Verification items for the finished model (mm, model axes). A direction names the side the tool comes from. Give positions to 0.01 mm unless a question says otherwise; leave off trailing zeros. Order: outer loops, then holes, each group sorted by start corner. A loop starts at its lowest first (then second) coordinate and runs counter-clockwise, first axis right, second up.
from build123d import *

# Parameters (mm, degrees)
SKETCH1_W                                     = 230
SKETCH1_H                                     = 123
SKETCH1_W_2                                   = 206
SKETCH1_H_2                                   = 99
BOSS_EXTRUDE1_DEPTH                           = 4
SKETCH2_W                                     = 230
SKETCH2_H                                     = 4
BOSS_EXTRUDE2_DEPTH                           = 6
BOSS_EXTRUDE3_DEPTH                           = 5
FILLET1_R                                     = 15
BOSS_EXTRUDE4_DEPTH                           = 4
FILLET2_R                                     = 5
FILLET3_R                                     = 3
CSK_FOR_4_FLAT_HEAD_MACHINE_SCREW1_AT_2_COUNT = 2
CSK_FOR_4_FLAT_HEAD_MACHINE_SCREW1_AT_2_PITCH = 30
CSK_FOR_4_FLAT_HEAD_MACHINE_SCREW1_AT_3_COUNT = 2
CSK_FOR_4_FLAT_HEAD_MACHINE_SCREW1_AT_3_PITCH = 225.008888713
CSK_FOR_4_FLAT_HEAD_MACHINE_SCREW1_AT_4_COUNT = 2
CSK_FOR_4_FLAT_HEAD_MACHINE_SCREW1_AT_4_PITCH = 223


with BuildPart() as part:
    # Sketch1 → Boss-Extrude1 (new body)
    with BuildSketch(Plane.XY):
        Rectangle(SKETCH1_W, SKETCH1_H)
        Rectangle(SKETCH1_W_2, SKETCH1_H_2, mode=Mode.SUBTRACT)
    extrude(amount=BOSS_EXTRUDE1_DEPTH)

    # Sketch2 → Boss-Extrude2 (add)
    with BuildSketch(Plane(origin=(0, 61.5, 0), x_dir=(1, 0, 0), z_dir=(0, 1, 0))):
        Polygon((-115, 10), (-115, 0), (115, 0), (115, 10), (115, 93), (105, 93), (105, 10), (-105, 10), (-105, 93), (-115, 93), align=None)
        with Locations((0, -2)):
            Rectangle(SKETCH2_W, SKETCH2_H)
    boss_extrude2 = extrude(amount=BOSS_EXTRUDE2_DEPTH)

    # Mirror1: Boss-Extrude2 across plane
    add(boss_extrude2.mirror(Plane.ZX))

    # Sketch3 → Boss-Extrude3 (add)
    with BuildSketch(Plane.ZY.offset(115)):
        Polygon((-93, 61.5), (0, 61.5), (0, -61.5), (-93, -61.5), (-93, -67.5), (4, -67.5), (4, 67.5), (-93, 67.5), align=None)
        Polygon((0, 61.5), (-25, 61.5), (-21.666666667, 57.5), (0, 31.5), align=None)
        Polygon((0, -61.5), (0, -31.5), (-21.666666667, -57.5), (-25, -61.5), align=None)
        Polygon((-21.666666667, 57.5), (-25, 61.5), (-93, 61.5), (-93, 57.5), align=None)
        Polygon((-25, -61.5), (-21.666666667, -57.5), (-93, -57.5), (-93, -61.5), align=None)
    boss_extrude3 = extrude(amount=BOSS_EXTRUDE3_DEPTH)

    # Mirror2: Boss-Extrude3 across plane
    add(boss_extrude3.mirror(Plane(origin=(0, 0, 0), x_dir=(0, 0, 1), z_dir=(1, 0, 0))))

    # Fillet1
    fillet1_edges = [part.edges().sort_by_distance(p)[0] for p in [
        (117.5, 57.5, -21.666666667),
        (117.5, -57.5, -21.666666667),
        (117.5, -31.5, 0),
        (117.5, 31.5, 0),
        (-103, -49.5, 2),
        (103, -49.5, 2),
        (103, 49.5, 2),
        (-103, 49.5, 2),
        (105, 64.5, -10),
        (-105, 64.5, -10),
        (-105, -64.5, -10),
        (105, -64.5, -10),
        (-117.5, 57.5, -21.666666667),
        (-117.5, 31.5, 0),
        (-117.5, -31.5, 0),
        (-117.5, -57.5, -21.666666667),
    ]]
    fillet(fillet1_edges, radius=FILLET1_R)

    # Sketch4 → Boss-Extrude4 (add, symmetric)
    with BuildSketch(Plane(origin=(0, 0, 0), x_dir=(1, 0, 0), z_dir=(0, 1, 0))):
        Polygon((-120, 96.464101615), (-120, 0), (-116.5, 0), (-116.5, 90), (-110.5, 93.464101615), (-110.5, 96.464101615), align=None)
    extrude(amount=BOSS_EXTRUDE4_DEPTH, both=True)

    # Fillet2
    fillet2_edges = [part.edges().sort_by_distance(p)[0] for p in [
        (-118.25, 4, 0),
        (-118.25, -4, 0),
    ]]
    fillet(fillet2_edges, radius=FILLET2_R)

    # Fillet3
    fillet3_edges = [part.edges().sort_by_distance(p)[0] for p in [
        (120, 62.5, -93),
        (120, -62.5, -93),
        (105, 64.5, -93),
        (-120, 0, -96.464101615),
        (-105, 64.5, -93),
        (-105, -64.5, -93),
        (105, -64.5, -93),
        (-120, -62.5, -93),
        (-120, 62.5, -93),
    ]]
    fillet(fillet3_edges, radius=FILLET3_R)

    # Sketch6 → CSK for #4 Flat Head Machine Screw1 (revolve, cut)
    with BuildSketch(Plane(origin=(111.5, 61.5, -68), x_dir=(0, 0, -1), z_dir=(1, 0, 0))):
        Polygon((0, 0), (0, 6), (1.63195, 6), (1.63195, 2.409835609), (2.857501397, 1), (2.857501397, 0), align=None)
    csk_for_4_flat_head_machine_screw1 = revolve(axis=Axis((111.5, 55.15, -68), (0, 1, 0)), mode=Mode.SUBTRACT)

    # CSK for #4 Flat Head Machine Screw1 at 2: CSK for #4 Flat Head Machine Screw1 ×2
    with Locations(*[(0, 0, i * CSK_FOR_4_FLAT_HEAD_MACHINE_SCREW1_AT_2_PITCH) for i in range(1, CSK_FOR_4_FLAT_HEAD_MACHINE_SCREW1_AT_2_COUNT)]):
        add(csk_for_4_flat_head_machine_screw1, mode=Mode.SUBTRACT)

    # CSK for #4 Flat Head Machine Screw1 at 3: CSK for #4 Flat Head Machine Screw1 ×2
    with Locations(*[Vector(-0.9910719584243963, 0, 0.13332806615574816) * (i * CSK_FOR_4_FLAT_HEAD_MACHINE_SCREW1_AT_3_PITCH) for i in range(1, CSK_FOR_4_FLAT_HEAD_MACHINE_SCREW1_AT_3_COUNT)]):
        add(csk_for_4_flat_head_machine_screw1, mode=Mode.SUBTRACT)

    # CSK for #4 Flat Head Machine Screw1 at 4: CSK for #4 Flat Head Machine Screw1 ×2
    with Locations(*[(-i * CSK_FOR_4_FLAT_HEAD_MACHINE_SCREW1_AT_4_PITCH, 0, 0) for i in range(1, CSK_FOR_4_FLAT_HEAD_MACHINE_SCREW1_AT_4_COUNT)]):
        add(csk_for_4_flat_head_machine_screw1, mode=Mode.SUBTRACT)


solid = part.part
(1) Section check A-A, the plane y = -15. Enter the section's corners in (x, z), then the cut area to 3 significant figures.
Solved:
outline: (-120, 0) - (-103, 0) - (-103, 4) - (-120, 4) - close; (103, 0) - (120, 0) - (120, 4) - (103, 4) - close
area: 136 mm2
(2) Release check for a two-part mould opening along Z. For faces 1 (the cylindrical face through (-117.54, -56.12, -22.41)), 2 (the flat face through (120, 0, 2)), 3 (the flat face through (-113.54, 0.06, -91.71)), 4 (the cylindrical face through (114.035, 61.993, -69.319)) record: pulls with the +Z half, pulls with the -Z half, needs draft (parallel to the pull), parting line crosses it, or undercut.
Solved:
face 1: pulls with the -Z half
face 2: needs draft
face 3: undercut
face 4: undercut
(3) Go/stop test with flat-tipped pins: pin 1 (4 mm diameter, centred on x = 111.5, z = -38, fed in from +Y); pin 2 (6 mm diameter, centred on x = -9, y = -45, fed in from -Z) (3 decimals); pin 3 (0.9 mm diameter, centred on y = -1.5, z = -94.5, fed in from +X); pin 4 (6.5 mm diameter, centred on x = 40, y = -66, fed in from -Z). Record where each tip stops, or that it passes through.
Solved:
pin 1: stops at y = 67.5
pin 2: passes through
pin 3: stops at x = -110.5
pin 4: stops at z = -10
(4) Scan lines: line 1 (X direction, y = 65.5, z = -68); line 2 (Z direction, x = 111.5, y = 62.25); line 3 (Z direction, x = 111.5, y = 66.35). Record each from-to range of solid material in increasing order.
Solved:
line 1: x = -120 to -113.13, -109.87 to -105, 105 to 109.87, 113.13 to 120
line 2: z = -93 to -70.86, -65.14 to -40.86, -35.14 to 4
line 3: z = -93 to -69.63, -66.37 to -39.63, -36.37 to 4
(5) Section check B-B, the plane x = -59. Enter the section's corners in (y, z).
Solved:
outline: (-67.5, -10) - (-61.5, -10) - (-61.5, 0) - (-49.5, 0) - (-49.5, 4) - (-67.5, 4) - close; (49.5, 0) - (61.5, 0) - (61.5, -10) - (67.5, -10) - (67.5, 4) - (49.5, 4) - close
(6) Set-up check for faces 5 (the flat face through (-113, 64, -93)), 6 (the cylindrical face through (117.54, -31.24, -0.92)), 7 (the cylindrical face through (100.72, 64.54, -14.51)), 8 (the cylindrical face through (-108.965, 61.993, -39.319)), 9 (the cylindrical face through (-98.72, 44.99, 2.03)): record each of +Z, -Z, +X, -X, +Y, -Y from which the full face is reachable in a straight line by a thin tool's end or side.
Solved:
face 5: -Z, +X, -X, +Y
face 6: -Z, +X, -X
face 7: -Z, +Y, -Y
face 8: none
face 9: +Z, -Z
(7) Section check C-C, the plane z = -75.5. Enter the section's corners in (x, y).
Solved:
outline: (-120, -67.5) - (-105, -67.5) - (-105, -61.5) - (-115, -61.5) - (-115, -57.5) - (-120, -57.5) - close; (-120, -4) - (-116.5, -4) - (-116.5, 4) - (-120, 4) - close; (-120, 57.5) - (-115, 57.5) - (-115, 61.5) - (-105, 61.5) - (-105, 67.5) - (-120, 67.5) - close; (105, -67.5) - (120, -67.5) - (120, -57.5) - (115, -57.5) - (115, -61.5) - (105, -61.5) - close; (105, 61.5) - (115, 61.5) - (115, 57.5) - (120, 57.5) - (120, 67.5) - (105, 67.5) - close
